```python
from build123d import *

# Parameters (mm, degrees)
BOSS_EXTRUDE1_DEPTH                 = 20.32
F_2_CLEARANCE_HOLE1_D               = 2.4384
F_2_CLEARANCE_HOLE1_DEPTH           = 7.62
F_2_CLEARANCE_HOLE1_TIP             = 0.732569267
TAP_DRILL_FOR_10_32_TAP1_D          = 4.0386
TAP_DRILL_FOR_10_32_TAP1_DEPTH      = 20.32
TAP_DRILL_FOR_10_32_TAP1_TIP        = 1.213317848
F_5_64_0_07813_DIAMETER_HOLE1_D     = 1.984502
F_5_64_0_07813_DIAMETER_HOLE1_DEPTH = 12.7
F_5_64_0_07813_DIAMETER_HOLE1_TIP   = 0.59620455
TAP_DRILL_FOR_6_32_TAP1_D           = 2.7051


with BuildPart() as part:
    # Sketch1 → Boss-Extrude1 (new body)
    with BuildSketch(Plane.XY):
        Polygon((0, 0), (25.4, 0), (29.21, 0), (29.21, 8.89), (22.86, 8.89), (22.86, 11.938), (20.32, 11.938), (20.32, 11.43), (0, 11.43), align=None)
    extrude(amount=BOSS_EXTRUDE1_DEPTH)

    # #2 Clearance Hole1
    with Locations(Plane(origin=(17.78, 11.43, 10.16), x_dir=(0, 0, 1), z_dir=(0, 1, 0))):
        with Locations((0, 0), (0, -3.81), (0, -7.62)):
            Hole(F_2_CLEARANCE_HOLE1_D / 2, depth=F_2_CLEARANCE_HOLE1_DEPTH)
            with Locations((0, 0, -(F_2_CLEARANCE_HOLE1_DEPTH + F_2_CLEARANCE_HOLE1_TIP / 2))):  # 118° drill point
                Cone(0, F_2_CLEARANCE_HOLE1_D / 2, F_2_CLEARANCE_HOLE1_TIP, mode=Mode.SUBTRACT)

    # Tap Drill for #10-32 Tap1
    with Locations(Plane(origin=(29.21, 3.81, 10.16), x_dir=(0, 1, 0), z_dir=(1, 0, 0))):
        with Locations((0, 0)):
            Hole(TAP_DRILL_FOR_10_32_TAP1_D / 2, depth=TAP_DRILL_FOR_10_32_TAP1_DEPTH)
            with Locations((0, 0, -(TAP_DRILL_FOR_10_32_TAP1_DEPTH + TAP_DRILL_FOR_10_32_TAP1_TIP / 2))):  # 118° drill point
                Cone(0, TAP_DRILL_FOR_10_32_TAP1_D / 2, TAP_DRILL_FOR_10_32_TAP1_TIP, mode=Mode.SUBTRACT)

    # 5/64 (0.07813) Diameter Hole1
    with Locations(Plane(origin=(0, 9.652, 6.35), x_dir=(0, 0, -1), z_dir=(-1, 0, 0))):
        with Locations((0, 0)):
            Hole(F_5_64_0_07813_DIAMETER_HOLE1_D / 2, depth=F_5_64_0_07813_DIAMETER_HOLE1_DEPTH)
            with Locations((0, 0, -(F_5_64_0_07813_DIAMETER_HOLE1_DEPTH + F_5_64_0_07813_DIAMETER_HOLE1_TIP / 2))):  # 118° drill point
                Cone(0, F_5_64_0_07813_DIAMETER_HOLE1_D / 2, F_5_64_0_07813_DIAMETER_HOLE1_TIP, mode=Mode.SUBTRACT)

    # Tap Drill for #6-32 Tap1 (through all)
    with Locations(Plane(origin=(26.035, 8.89, 17.145), x_dir=(0, 0, 1), z_dir=(0, 1, 0))):
        with Locations((0, 0), (-13.97, 0)):
            Hole(TAP_DRILL_FOR_6_32_TAP1_D / 2)


solid = part.part
```
Read the model definition and answer for the solid it produces. Units are mm, in the model's axes. A direction names the side the tool comes from. Coordinates: 2 decimals unless noted, no trailing zeros. Loops run counter-clockwise (first coordinate to the right, second up) from the corner with the lowest first, then second, coordinate; pieces in that order, holes last.
(1) Flat-ended cylindrical pins translate along their axes: pin 1 Ø2 at (x, z) = (5, 17) entering from +Y; pin 2 Ø1.9 at (x, z) = (24.5, 9) entering from +Y; pin 3 Ø2.5 at (x, z) = (26.035, 3.175) entering from -Y; pin 4 Ø3.5 at (y, z) = (3.81, 10.16) entering from +X. Find the tip coordinate at first contact, or state that the pin passes through.
Solution:
pin 1: stops at y = 11.43
pin 2: stops at y = 8.89
pin 3: passes through
pin 4: stops at x = 8.73
(2) A tool of negligible diameter and unlimited length cuts with its end or side. For faces 1 (the face through (17.83, 8.38, 11.38)), 2 (the face through (8, 11.43, 10)), 3 (the face through (22.86, 10, 10)), 4 (the face through (18.908, 1.945, 9.387)), from which of +Z, -Z, +X, -X, +Y, -Y can it reach the whole face along a straight path? Write none if from no direction.
Solution:
face 1: +Y
face 2: +Z, -Z, -X, +Y
face 3: +Z, -Z, +X, +Y
face 4: +X
(3) The part is cut by section D-D (x = 9.25). Determine the outline of the cut face in (y, z), and give its area (3 significant figures).
Solution:
outline: (0, 0) - (11.43, 0) - (11.43, 9.35) - (5.66, 9.35) arc R2.02 cw (long way) to (5.66, 10.97) - (11.43, 10.97) - (11.43, 20.32) - (0, 20.32) - close; hole circle Ø1.98 at (9.65, 6.35)
area: 207 mm2
(4) The part is cut by section B-B (x = 13.97). Determine the outline of the cut face in (y, z), and give its area (3 significant figures).
Solution:
outline: (0, 0) - (11.43, 0) - (11.43, 8.94) - (5.42, 8.94) arc R2.02 cw (long way) to (5.42, 11.38) - (11.43, 11.38) - (11.43, 20.32) - (0, 20.32) - close
area: 205 mm2
(5) The part is cut by section A-A (z = 2.25). Determine the outline of the cut face in (x, y), and give its area (3 significant figures).
Solution:
outline: (0, 0) - (25.05, 0) - (25.05, 8.89) - (22.86, 8.89) - (22.86, 11.94) - (20.32, 11.94) - (20.32, 11.43) - (0, 11.43) - close; (27.02, 0) - (29.21, 0) - (29.21, 8.89) - (27.02, 8.89) - close
area: 301 mm2
(6) The part is cut by section C-C (z = 19.25). Determine the outline of the cut face in (x, y).
Solution:
outline: (0, 0) - (29.21, 0) - (29.21, 8.89) - (22.86, 8.89) - (22.86, 11.94) - (20.32, 11.94) - (20.32, 11.43) - (0, 11.43) - close
(7) The mould has two halves that part along Y. Classify faces 5 (the face through (26, 8.89, 10)), 6 (the face through (7.887, 3.734, 9.818)), 7 (the face through (29.21, 6, 10)): released by +Y, released by -Y, zero draft, split by the parting line, or undercut.
Solution:
face 5: released by +Y
face 6: undercut
face 7: zero draft
(8) Consider line 1 along X through (y, z) = (6.5, 10.16); line 2 along Z through (x, y) = (17.78, 7.25); line 3 along Y through (x, z) = (7, 6.35). Determine where each line is inside the solid, lowest interval first.
Solution:
line 1: x = 0 to 8.94, 11.38 to 12.75, 15.19 to 16.56, 19 to 29.21
line 2: z = 0 to 8.94, 11.38 to 20.32
line 3: y = 0 to 8.66, 10.64 to 11.43
